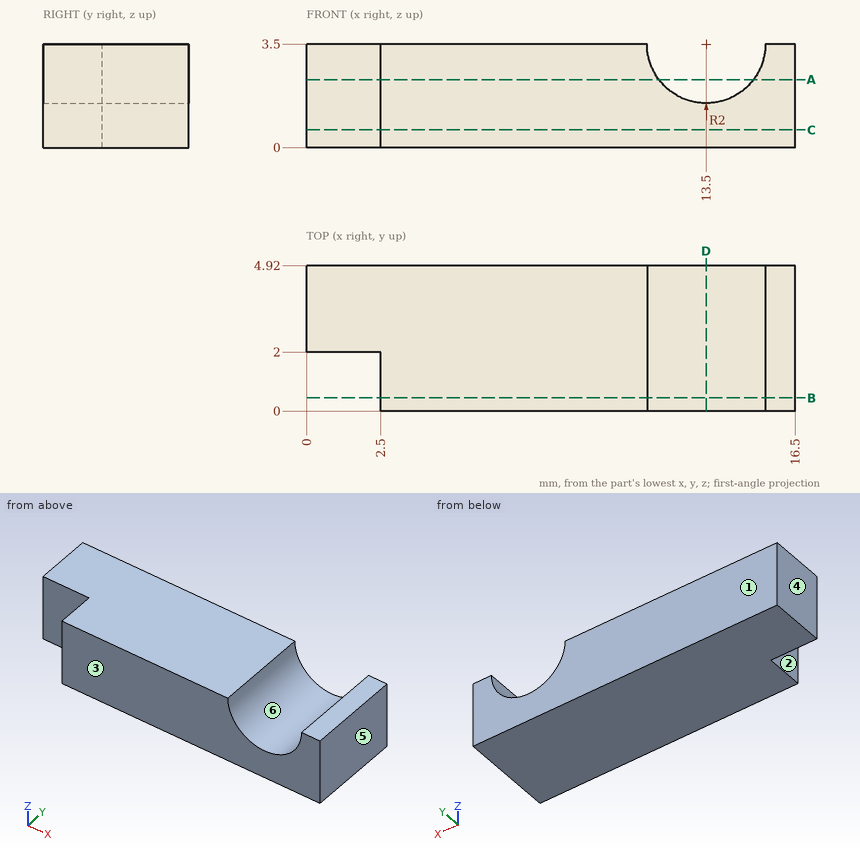
Geometry check sheet. Reference: drawing and pictorial views, mm from the part's lowest x, y, z. A direction names the side the tool comes from. Round coordinates to 2 decimals unless told otherwise and drop trailing zeros. Order: outer loops, then holes, each group sorted by start corner. A loop starts at its lowest first (then second) coordinate and runs counter-clockwise, first axis right, second up. Notation, with made-up numbers: M -16,74.5 L 0,74.5 A7 ccw 0,82.5 Z; hole C 83.25,-3.75 d8. An arc over 180 degrees is marked long. Answer as CSV lines item,"result".
1) Sectioned sample at C-C on z = 0.6. Record the cut outline in (x, y), and give its area (3 significant figures).
Entries:
outline,"M 0,2 L 2.5,2 L 2.5,0 L 16.5,0 L 16.5,4.92 L 0,4.92 Z"
area,"76.2 mm2"
2) Sectioned sample at A-A on z = 2.3. Record the cut outline in (x, y).
Entries:
outline,"M 0,2 L 2.5,2 L 2.5,0 L 11.9,0 L 11.9,4.92 L 0,4.92 Z; M 15.1,0 L 16.5,0 L 16.5,4.92 L 15.1,4.92 Z"
3) Tool access check on the marked faces 1 and 2. Record the directions out of +Z, -Z, +X, -X, +Y, -Y that give a thin tool (end or side, any length) a straight path to the whole face; none if there is none.
Entries:
face 1,"+Z, -Z, +X, -X, +Y"
face 2,"+Z, -Z, -X, -Y"
4) Sectioned sample at D-D on x = 13.5. Record the cut outline in (y, z), and give its area (3 significant figures).
Entries:
outline,"M 0,0 L 4.92,0 L 4.92,1.5 L 0,1.5 Z"
area,"7.38 mm2"
5) Sectioned sample at B-B on y = 0.45. Record the cut outline in (x, z).
Entries:
outline,"M 2.5,0 L 16.5,0 L 16.5,3.5 L 15.5,3.5 A2 cw 11.5,3.5 L 2.5,3.5 Z"
6) Thickness scan on probe 1 along Y at (x, z) = (0.75, 0.2); probe 2 along X at (y, z) = (4.25, 1.9); probe 3 along X at (y, z) = (0.6, 1.9). Record the ranges inside material, lowest first. Write a range as [from, to].
Entries:
probe 1,"[2, 4.92]"
probe 2,"[0, 12.3], [14.7, 16.5]"
probe 3,"[2.5, 12.3], [14.7, 16.5]"
7) Gauge pin test, flat end, axial feed: pin 1 Ø0.6 at (y, z) = (1, 2.5) entering from -X. Record the tip position at first contact, or that the pin passes through.
Entries:
pin 1,"x = 2.5"
8) Mould release check, pull along X, two halves, no side actions. Record for the marked faces 3, 4, 5 and 6: +X half, -X half, draft (parallel to the pull), parting line (faces both ways), or undercut.
Entries:
face 3,"draft"
face 4,"-X half"
face 5,"+X half"
face 6,"undercut"
